Design review of the part built by this model. Coordinates are the model's own, in mm. Face numbers are marked on the shaded views. A direction names the side the tool comes from. Round coordinates to 2 decimals unless told otherwise and drop trailing zeros. Order: outer loops, then holes, each group sorted by start corner. A loop starts at its lowest first (then second) coordinate and runs counter-clockwise, first axis right, second up. Notation, with made-up numbers: (5.25, 72.25) - (28.25, 72.25) arc R26 cw to (28.25, 89.25) - close; hole circle Ø7 at (1.5, -21). An arc over 180 degrees is marked (long way). Use CSV: the item, a comma, the result in double quotes. Start each with the question number.
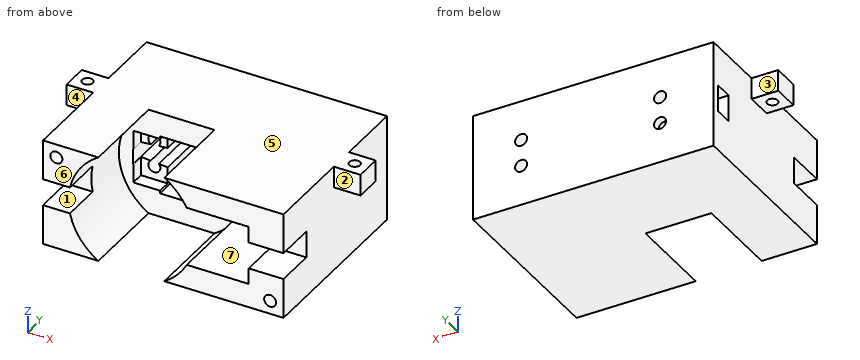
Solid Edge part; units mm, degrees
sketch "Sketch1" plane through (0, 0, 0) normal (0, -1, 0) x (1, 0, 0)
  line L0 (31.4924, 49.0939) -> (121.4924, 49.0939)
  line L1 (121.4924, 49.0939) -> (121.4924, 9.0939)
  line L2 (121.4924, 9.0939) -> (31.4924, 9.0939)
  line L3 (31.4924, 9.0939) -> (31.4924, 49.0939)
  dimension "D1" = 31.4924
  dimension "D2" = 121.4924
extrude "Protrusion1" add sketch "Sketch1" against normal blind 40
sketch "Sketch2" plane through (64.4924, 0, 22.0939) normal (0, -1, 0) x (1, 0, 0)
  line L0 (-18.0616, 9.8803) -> (-8, 10.7605)
  line L1 (-8, 10.7605) -> (-8, 18.0605)
  line L2 (-8, 18.0605) -> (34, 18.0605)
  line L3 (34, -4) -> (34, 18.0605)
  line L4 (-8, -4) -> (34, -4)
  line L5 (-8, -4) -> (-8, 3.3)
  line L6 (-8, 3.3) -> (-18.0616, 4.1803)
  line L7 (-18.0616, 4.1803) -> (-18.0616, 9.8803)
extrude "ExtrudedCutout_4" cut sketch "Sketch2" against normal blind 37
sketch "Sketch3" plane through (31.4924, 20, 22.0939) normal (-1, 0, 0) x (0, -1, 0)
  line L0 (-17, 2) -> (-17, 12)
  line L1 (-17, 12) -> (-10, 12)
  line L2 (-10, 12) -> (-10, 2)
  line L3 (-10, 2) -> (-17, 2)
  dimension "D1" = 17
  dimension "D2" = 17
  dimension "D3" = 10
extrude "Cutout1" cut sketch "Sketch3" against normal up to next
sketch "Sketch4" plane through (64.4924, 0, 22.0939) normal (0, -1, 0) x (1, 0, 0)
  line L0 (-8, 17.0605) -> (-18, 17.0605)
  line L1 (-18, 17.0605) -> (-18, -2.9395)
  line L2 (-18, -2.9395) -> (-8, -2.9395)
  line L3 (-8, -2.9395) -> (-8, 17.0605)
  line L4 (34, 17.0605) -> (44, 17.0605)
  line L5 (44, 17.0605) -> (44, -2.9395)
  line L6 (44, -2.9395) -> (34, -2.9395)
  line L7 (34, -2.9395) -> (34, 17.0605)
  dimension "D1" = 44
  dimension "D2" = 8
  dimension "D3" = 18
  dimension "D4" = 34
extrude "ExtrudedCutout_6" cut sketch "Sketch4" against normal blind 10
sketch "Sketch5" plane through (91.2324, 10, 21.645) normal (0, -1, 0) x (1, 0, 0)
  circle A0 centre (12.26, 12.5095) radius 1.65
  circle A1 centre (-39.74, 12.5095) radius 1.65
  circle A2 centre (-39.74, 2.5095) radius 1.65
  circle A3 centre (12.26, 2.5095) radius 1.65
  dimension "D1" = 39.74
  dimension "D2" = 12.26
  dimension "D3" = 39.74
extrude "Cutout2" cut sketch "Sketch5" against normal through all
sketch "Sketch6" plane through (64.4924, 0, 22.0939) normal (0, -1, 0) x (1, 0, 0)
  circle A0 centre (39, 2.0605) radius 2.25
  circle A1 centre (-13, 12.0605) radius 2.25
  circle A2 centre (-13, 2.0605) radius 2.25
  circle A3 centre (39, 12.0605) radius 2.25
extrude "Cutout3" cut sketch "Sketch6" against normal up to next
sketch "Sketch7" plane through (68.9924, 0, 22.0939) normal (0, -1, 0) x (1, 0, 0)
  line L0 (-37.5, 27) -> (-37.5, -13)
  line L1 (-37.5, -13) -> (52.5, -13)
  line L2 (52.5, -13) -> (52.5, 27)
  line L3 (52.5, 27) -> (-37.5, 27)
  line L4 (-22.5616, 13.0605) -> (-22.5616, 18.0605)
  line L5 (-22.5616, 18.0605) -> (39.5, 18.0605)
  line L6 (39.5, 18.0605) -> (39.5, -4)
  line L7 (39.5, -4) -> (-22.5616, -4)
  line L8 (-22.5616, 13.0605) -> (-22.5616, -4)
  dimension "D1" = 39.5
extrude "ExtrudedProtrusion_4" add sketch "Sketch7" along normal blind 28.07
sketch "Sketch8" plane through (68.9924, -28.07, 22.0939) normal (0, -1, 0) x (1, 0, 0)
  circle A0 centre (-4.46, 7) radius 23.5
extrude "ExtrudedCutout_9" cut sketch "Sketch8" against normal blind 33.07
sketch "Sketch9" plane through (41.8429, -28.07, 29.0939) normal (0, -1, 0) x (0, 0, 1)
  line L0 (0, 10.3505) -> (5, 10.3505)
  line L1 (5, 10.3505) -> (5, -79.6495)
  line L2 (5, -79.6495) -> (0, -79.6495)
  line L3 (0, -79.6495) -> (-5, -79.6495)
  line L4 (-5, -79.6495) -> (-5, 10.3505)
  line L5 (-5, 10.3505) -> (0, 10.3505)
  dimension "D1" = 5
extrude "Cutout4" cut sketch "Sketch9" against normal blind 15
sketch "Sketch10" plane through (41.8429, -28.07, 41.5939) normal (0, -1, 0) x (0, 0, 1)
  circle A0 centre (2.5, 5.3505) radius 2.25
  circle A1 centre (-27.5, -74.6495) radius 2.25
  dimension "D1" = 2.5
extrude "ExtrudedCutout_13" cut sketch "Sketch10" against normal blind 5
sketch "Sketch11" plane through (76.4924, 5.965, 49.0939) normal (0, 0, 1) x (-1, 0, 0)
  line L0 (-0.379, 0.965) -> (24.299, 0.965)
  line L1 (24.299, 0.965) -> (45, 0.965)
  line L2 (45, 0.965) -> (55, 0.965)
  line L3 (55, 0.965) -> (55, -9.035)
  line L4 (55, -9.035) -> (45, -9.035)
  line L5 (45, -9.035) -> (-45, -9.035)
  line L6 (-45, -9.035) -> (-55, -9.035)
  line L7 (-55, -9.035) -> (-55, 0.965)
  line L8 (-55, 0.965) -> (-45, 0.965)
  line L9 (-45, 0.965) -> (-0.379, 0.965)
  dimension "D1" = 55
  dimension "D2" = 45
  dimension "D3" = 45
  dimension "D4" = 55
extrude "ExtrudedProtrusion_9" add sketch "Sketch11" against normal blind 8
sketch "Sketch12" plane through (26.4924, 10, 41.0939) normal (0, 0, -1) x (-1, 0, 0)
  circle A0 centre (0, 0) radius 2
  circle A1 centre (-100, 0) radius 2
extrude "Cutout5" cut sketch "Sketch12" against normal through all
Q1. Clearance check with flat-ended pins moving along their axes: pin 1 (3 mm diameter, centred on y = 18.5, z = 44.5, fed in from -X); pin 2 (8 mm diameter, centred on x = 115.5, z = 30.5, fed in from -Y); pin 3 (4 mm diameter, centred on x = 28.5, z = 43.5, fed in from +Y); pin 4 (3 mm diameter, centred on y = -13.5, z = 28, fed in from +X). State where each tip first meets the part, or that it passes through.
Q2. Tool access review of the marked faces 1, 2, 3 and 4: name each direction out of +Z, -Z, +X, -X, +Y, -Y from which nothing blocks a thin tool from reaching the whole face with its end or side.
Q3. Take a section at B-B (z = 15). State the section outline as (x, y) points.
Q4. For L1, parallel to X at y = 0, z = 29; L2, parallel to Z at x = 94, y = 26; L3, parallel to X at y = 0, z = 24, list the stretches that pass through material, from the lowest coordinate up. Write a range as [from, to].
Q5. Take a section at A-A (x = 63). State the section outline as (y, z) points, plus the area to 3 significant figures.
Q6. The part is to be moulded in two halves that separate along Z. For the marked faces 5, 6 and 7, say which applies: +Z half, -Z half, draft (parallel to the pull), parting line (faces both ways), or undercut.
Findings below:
1,pin 1,"stops at x = 31.49"
1,pin 2,"stops at y = -28.07"
1,pin 3,"stops at y = 15"
1,pin 4,"stops at x = 121.49"
2,face 1,"+X, -X, -Y"
2,face 2,"+Z, -Z, +X, -Y"
2,face 3,"+Z, -Z, -X, +Y"
2,face 4,"+Z, -Z, -X, -Y"
3,outline,"(31.49, -28.07) - (45.73, -28.07) - (45.73, 5) - (83.34, 5) - (83.34, -28.07) - (114.43, -28.07) - (114.43, -23.07) - (118.55, -23.07) - (118.55, -28.07) - (121.49, -28.07) - (121.49, 40) - (31.49, 40) - close"
4,L1,"x = [31.49, 41.03], [108.49, 121.49]"
4,L2,"z = [9.09, 18.09], [40.15, 49.09]"
4,L3,"x = [31.49, 41.59], [108.49, 121.49]"
5,outline,"(5, 9.09) - (40, 9.09) - (40, 49.09) - (5, 49.09) - (5, 40.15) - (37, 40.15) - (37, 18.09) - (5, 18.09) - close"
5,area,"694 mm^2"
6,face 5,"+Z half"
6,face 6,"draft"
6,face 7,"undercut"
